Study the drawing (mm; zero at the part's minimum x, y, z) and answer. Give positions to 0.01 mm unless a question says otherwise; leave off trailing zeros. Loops run counter-clockwise (first coordinate to the right, second up) from the corner with the lowest first, then second, coordinate; pieces in that order, holes last. Notation, with made-up numbers: (75, 35) - (108, 35) arc R14 ccw to (108, 61) - close; hole circle Ø4 at (18, 36.25). An arc over 180 degrees is marked (long way). Write item = value, one per line. Start each with the question number.
1) Flat-ended cylindrical pins translate along their axes: P1, Ø0.6, axis at y = 0.5, z = 6, coming from the +X side; P2, Ø0.6, axis at x = 88, y = 1, coming from the -Z side. Find the tip coordinate at first contact, or state that the pin passes through.
2) The part is cut by section A-A on x = 31.5. Write down the section's boundary in (y, z), plus the area to 3 significant figures.
3) Consider probe 1 along Z at (x, y) = (47.5, 0.7); probe 2 along X at (y, z) = (0.2, 8.5). Determine where each line is inside the solid, lowest interval first.
4) The part is cut by section B-B on y = 0.6. Write down the section's boundary in (x, z), plus the area to 3 significant figures.
5) The part is cut by section C-C on z = 41. Write down the section's boundary in (x, y), plus the area to 3 significant figures.
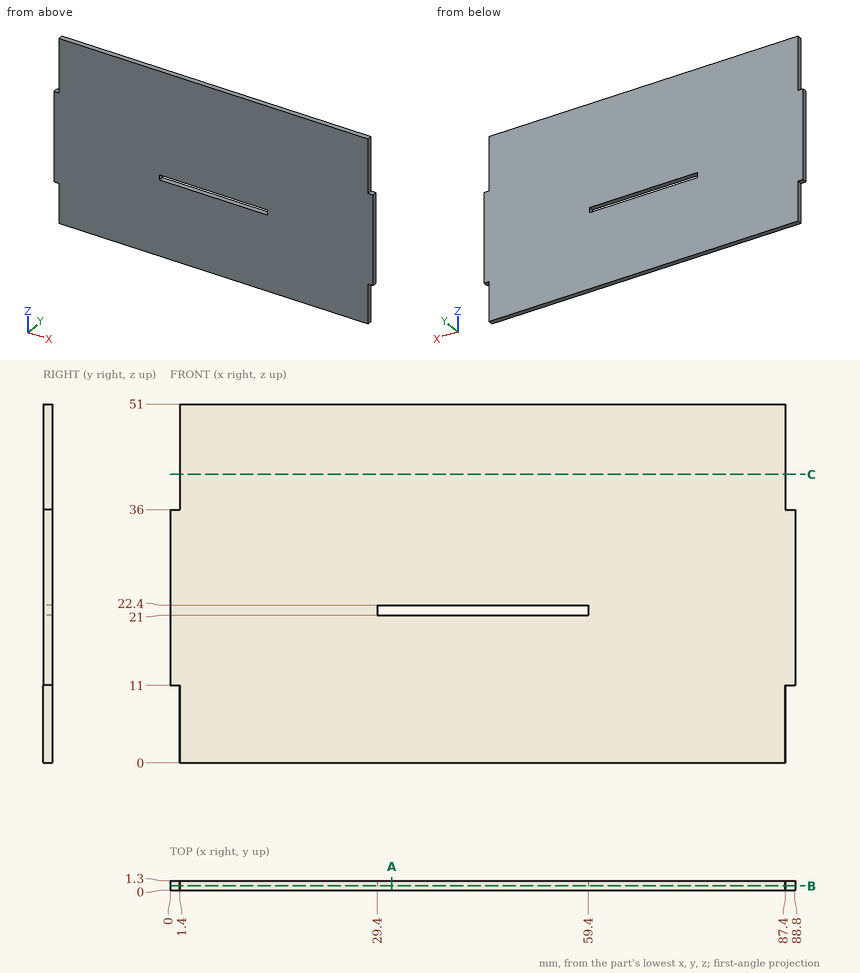
Answer below:
q1.P1 = 87.4
q1.P2 = 11
q2.outline = (0, 0) - (1.3, 0) - (1.3, 21) - (0, 21) - close; (0, 22.4) - (1.3, 22.4) - (1.3, 51) - (0, 51) - close
q2.area = 64.5 mm2
q3.probe_1 = 0 to 21, 22.4 to 51
q3.probe_2 = 1.4 to 87.4
q4.outline = (0, 11) - (1.4, 11) - (1.4, 0) - (87.4, 0) - (87.4, 11) - (88.8, 11) - (88.8, 36) - (87.4, 36) - (87.4, 51) - (1.4, 51) - (1.4, 36) - (0, 36) - close; hole (29.4, 21) - (59.4, 21) - (59.4, 22.4) - (29.4, 22.4) - close
q4.area = 4,410 mm2
q5.outline = (1.4, 0) - (87.4, 0) - (87.4, 1.3) - (1.4, 1.3) - close
q5.area = 112 mm2
